Source: CAD feature listing. Evaluate the final solid. Frame: model axes, mm. Give positions to 0.01 mm unless a question says otherwise; leave off trailing zeros. Loops run counter-clockwise (first coordinate to the right, second up) from the corner with the lowest first, then second, coordinate; pieces in that order, holes last.
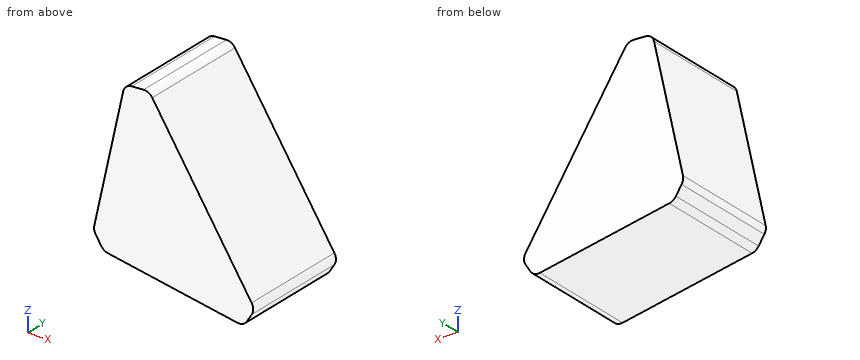
```python
from build123d import *

# Parameters (mm, degrees)
PAD018_DEPTH = 33
FILLET019_R  = 3
FILLET020_R  = 3


with BuildPart() as fillet020:
    # Sketch023 → Pad018 (new body)
    with BuildSketch(Plane(origin=(0, 0, 0), x_dir=(0.848048, 0, 0.529919), z_dir=(0, -1, 0))):
        Polygon((-40.765351, 19.72502), (-40.765351, 12.915253), (-0.082344, -5.035194), (5.261885, -2.605449), (20.317712, 40.085552), (14.098928, 44.660699), align=None)
    extrude(amount=PAD018_DEPTH)

    # Fillet019
    fillet019_edges = [fillet020.edges().sort_by_distance(p)[0] for p in [
        (-4.011709, -16.5, 44.761223),
        (-11.709995, -16.5, 45.345714),
    ]]
    fillet(fillet019_edges, radius=FILLET019_R)

    # Fillet020
    fillet020_edges = [fillet020.edges().sort_by_distance(p)[0] for p in [
        (5.843009, -16.5, 0.578828),
        (2.598414, -16.5, -4.313722),
        (-41.41502, -16.5, -10.649589),
        (-45.023647, -16.5, -4.874579),
    ]]
    fillet(fillet020_edges, radius=FILLET020_R)


with BuildPart() as part_mirroring015:
    # Part__Mirroring015: instance of Fillet020
    add(fillet020.part.mirror(Plane(origin=(0, 0, 0), x_dir=(0, -1, 0), z_dir=(1, 0, 0))))


with BuildPart() as part_mirroring015_1:
    # Part__Mirroring015 placement: moved
    add(part_mirroring015.part.moved(Location((76, 0, 0))))


solid = part_mirroring015_1.part
```
(1) Ray query, line 1 along X through (y, z) = (-9, 20.5); line 2 along Z through (x, y) = (92, -30.5); line 3 along X through (y, z) = (-20.5, 38). Return the intervals inside material, ascending.
A:
line 1: x = 74.6 to 104.19
line 2: z = -6.99 to 38.88
line 3: x = 78.5 to 92.58
(2) Section A-A, the plane y = -17. Return the cut outline in (x, z), then the cut area to 3 significant figures.
A:
outline: (70.44, 1.83) arc R3 ccw to (70.86, -0.49) - (72.66, -3.19) arc R3 ccw to (74.73, -4.51) - (115.48, -10.37) arc R3 ccw to (118.45, -8.99) - (120, -6.51) arc R3 ccw to (119.96, -3.26) - (88.68, 43.88) arc R3 ccw to (85.96, 45.21) - (82.23, 44.93) arc R3 ccw to (79.53, 42.59) - close
area: 1,600 mm2
(3) First-contact query: pin 1 (1 mm diameter, centred on y = -18.5, z = 9.5, fed in from -X); pin 2 (1 mm diameter, centred on y = -7.5, z = 29.5, fed in from +X); pin 3 (5 mm diameter, centred on x = 108.5, z = 19, fed in from -Y); pin 4 (4 mm diameter, centred on x = 102.5, y = -18.5, fed in from -Z). Flat tips, straight axial feed; report the tip coordinate or a pass-through.
A:
pin 1: stops at x = 72.04
pin 2: stops at x = 98.55
pin 3: passes through
pin 4: stops at z = -8.79
(4) Section B-B, the plane x = 90. Return the cut outline in (y, z), then the cut area to 3 significant figures.
A:
outline: (-33, -6.7) - (0, -6.7) - (0, 41.89) - (-33, 41.89) - close
area: 1,600 mm2
(5) Section C-C, the plane z = 0.5. Return the cut outline in (x, y), then the cut area to 3 significant figures.
A:
outline: (70.44, -33) - (117.46, -33) - (117.46, 0) - (70.44, 0) - close
area: 1,550 mm2
